from build123d import *

# Parameters (mm, degrees)
EXTRUDE_1_DEPTH     = 10
SKETCH_2_R          = 1.5
CUT_EXTRUDE_1_DEPTH = 10


with BuildPart() as part:
    # 草图1 → 凸台-拉伸1 (new body)
    with BuildSketch(Plane.XY):
        with BuildLine():
            Line((-20, 1.5), (-20, 3))
            Line((-20, 3), (-15.766281297, 3))
            ThreePointArc((-15.766281297, 3), (-10.6923358, 6.463023375), (-5, 4.153311931))
            ThreePointArc((-5, 4.153311931), (0, 6.5), (5, 4.153311931))
            ThreePointArc((5, 4.153311931), (10.6923358, 6.463023375), (15.766281297, 3))
            Line((15.766281297, 3), (20, 3))
            Line((20, 3), (20, 1.5))
            Line((20, 1.5), (14.769696007, 1.5))
            ThreePointArc((14.769696007, 1.5), (10, 5), (5.230303993, 1.5))
            Line((5.230303993, 1.5), (4.769696007, 1.5))
            ThreePointArc((4.769696007, 1.5), (0, 5), (-4.769696007, 1.5))
            Line((-4.769696007, 1.5), (-5.230303993, 1.5))
            ThreePointArc((-5.230303993, 1.5), (-10, 5), (-14.769696007, 1.5))
            Line((-14.769696007, 1.5), (-20, 1.5))
        make_face()
    extrude(amount=EXTRUDE_1_DEPTH)

    # 草图2 → 切除-拉伸1 (cut)
    with BuildSketch(Plane(origin=(0, 3, 0), x_dir=(1, 0, 0), z_dir=(0, 1, 0))):
        with Locations(Location((-18, -3, 0), (0, 0, 270))):
            Circle(SKETCH_2_R)
        with Locations(Location((-18, -7, 0), (0, 0, 180))):
            Circle(SKETCH_2_R)
        with Locations(Location((18, -7, 0), (0, 0, 270))):
            Circle(SKETCH_2_R)
        with Locations(Location((18, -3, 0), (0, 0, 180))):
            Circle(SKETCH_2_R)
    extrude(amount=-CUT_EXTRUDE_1_DEPTH, mode=Mode.SUBTRACT)


solid = part.part
The model under review builds one solid part; all positions refer to its coordinate system, in mm. A direction names the side the tool comes from. Round coordinates to 2 decimals unless told otherwise and drop trailing zeros. Order: outer loops, then holes, each group sorted by start corner. A loop starts at its lowest first (then second) coordinate and runs counter-clockwise, first axis right, second up. Notation, with made-up numbers: (-9.75, 36) -> (39.25, 36) arc R4 ccw to (39.25, 41) -> close; hole circle Ø11 at (-10, 66). An arc over 180 degrees is marked (long way). Write item = value, one per line. Start each with the question number.
Item 1: For line 1 along X through (y, z) = (4.6, 3); line 2 along X through (y, z) = (3.85, 7); line 3 along X through (y, z) = (2.95, 4.25), list the stretches that pass through material, from the lowest coordinate up.
Item 2: Consider section B-B on z = 3. Write out the cut boundary in (x, y).
Item 3: Clearance check with flat-ended pins moving along their axes: pin 1 Ø1.5 at (x, z) = (-9.5, 5) entering from -Y; pin 2 Ø3 at (x, z) = (-14.5, 5.5) entering from -Y; pin 3 Ø1.8 at (x, z) = (18, 3) entering from +Y; pin 4 Ø6 at (x, z) = (9, 6.5) entering from -Y. State where each tip first meets the part, or that it passes through.
Item 4: Mouldability with a two-part tool opening along Z and no side actions: class faces 3 (the face through (-18, 3, 5)), 4 (the face through (0.28, 5.15, 10)), 5 (the face through (19.01, 2.26, 5.89)), 6 (the face through (19.5, 2.26, 3.07)) as released by +Z, released by -Z, zero draft, split by the parting line, or undercut.
Item 5: Consider section D-D on z = 6.5. Write out the cut boundary in (x, y), plus the area to 3 significant figures.
Item 6: For faces 1 (the face through (18, 3, 5)), 2 (the face through (20, 2, 5)), list the 3-axis set-ups (+Z, -Z, +X, -X, +Y, -Y) from which the entire face can be reached by the end or side of a thin tool; tool diameter is ignored.
Item 7: Consider section A-A on x = -18. Write out the cut boundary in (y, z).
Item 8: Consider section C-C on y = 3.55. Write out the cut boundary in (x, z).
Conclusion:
q1.line_1 = -14.59 to -11.96, -8.04 to -5.41, -4.59 to -1.96, 1.96 to 4.59, 5.41 to 8.04, 11.96 to 14.59
q1.line_2 = -15.24 to -13.19, -6.81 to -3.19, 3.19 to 6.81, 13.19 to 15.24
q1.line_3 = -20 to -18.83, -17.17 to -14.04, -5.96 to -4.04, 4.04 to 5.96, 14.04 to 17.17, 18.83 to 20
q2.outline = (-20, 1.5) -> (-19.5, 1.5) -> (-19.5, 3) -> (-20, 3) -> close; (-16.5, 1.5) -> (-14.77, 1.5) arc R5 cw to (-5.23, 1.5) -> (-4.77, 1.5) arc R5 cw to (4.77, 1.5) -> (5.23, 1.5) arc R5 cw to (14.77, 1.5) -> (16.5, 1.5) -> (16.5, 3) -> (15.77, 3) arc R6.5 ccw to (5, 4.15) arc R6.5 ccw to (-5, 4.15) arc R6.5 ccw to (-15.77, 3) -> (-16.5, 3) -> close; (19.5, 1.5) -> (20, 1.5) -> (20, 3) -> (19.5, 3) -> close
q3.pin_1 = 4.84
q3.pin_2 = 1.5
q3.pin_3 = through
q3.pin_4 = 3
q4.face_3 = zero draft
q4.face_4 = released by +Z
q4.face_5 = undercut
q4.face_6 = undercut
q5.outline = (-20, 1.5) -> (-19.41, 1.5) -> (-19.41, 3) -> (-20, 3) -> close; (-16.59, 1.5) -> (-14.77, 1.5) arc R5 cw to (-5.23, 1.5) -> (-4.77, 1.5) arc R5 cw to (4.77, 1.5) -> (5.23, 1.5) arc R5 cw to (14.77, 1.5) -> (16.59, 1.5) -> (16.59, 3) -> (15.77, 3) arc R6.5 ccw to (5, 4.15) arc R6.5 ccw to (-5, 4.15) arc R6.5 ccw to (-15.77, 3) -> (-16.59, 3) -> close; (19.41, 1.5) -> (20, 1.5) -> (20, 3) -> (19.41, 3) -> close
q5.area = 62.5 mm2
q6.face_1 = +Z, -Z, +X, +Y
q6.face_2 = +Z, -Z, +X, +Y, -Y
q7.outline = (1.5, 0) -> (3, 0) -> (3, 1.5) -> (1.5, 1.5) -> close; (1.5, 4.5) -> (3, 4.5) -> (3, 5.5) -> (1.5, 5.5) -> close; (1.5, 8.5) -> (3, 8.5) -> (3, 10) -> (1.5, 10) -> close
q8.outline = (-15.44, 0) -> (-13.52, 0) -> (-13.52, 10) -> (-15.44, 10) -> close; (-6.48, 0) -> (-3.52, 0) -> (-3.52, 10) -> (-6.48, 10) -> close; (3.52, 0) -> (6.48, 0) -> (6.48, 10) -> (3.52, 10) -> close; (13.52, 0) -> (15.44, 0) -> (15.44, 10) -> (13.52, 10) -> close
